Input: part model. Units: mm. Frame: model coordinates. Face numbers are marked on the shaded views. Coordinates: 2 decimals unless noted, no trailing zeros. Loops run counter-clockwise (first coordinate to the right, second up) from the corner with the lowest first, then second, coordinate; pieces in that order, holes last. Notation, with made-up numbers: M -32.5,16 L -4.5,16 A30 ccw -4.5,40 Z; hole C 4,44.25 d6. An arc over 180 degrees is marked long. Use a Markdown table: item, result. Add a question column.
1. Section A-A on z = -31.5. Output: boundary loops of the cut face in (x, y).
2. Line query: L1, parallel to Z at x = 0, y = -244.85; L2, parallel to Z at x = 96, y = -150; L3, parallel to X at y = -150, z = -8. Output: solid intervals per line, ascending. Write a range as [from, to].
3. Draft query along Y for the marked faces 1 and 2. Return one class per face: +Y half, -Y half, draft (parallel to the pull), parting line (faces both ways), or undercut.
4. Pin query (flat end, axial travel): pin 1 (1.5 mm diameter, centred on y = -114.5, z = -52.5, fed in from +X); pin 2 (10 mm diameter, centred on y = -105, z = -14, fed in from -X); pin 3 (3.5 mm diameter, centred on y = -150, z = 8, fed in from +X); pin 4 (3 mm diameter, centred on x = -8, z = -43, fed in from -Y). Return the tip coordinate at first contact, or that it passes through.
```python
from build123d import *

# Parameters (mm, degrees)
SKETCH051_R                 = 2.8
EXTRUDE033_DEPTH            = 20
CYLINDER153_R               = 2.13
CYLINDER153_DEPTH           = 300
CYLINDER154_R               = 2.13
CYLINDER154_DEPTH           = 300
TUBE008_R                   = 98
TUBE008_R_2                 = 94
TUBE008_DEPTH               = 65
SKETCH050_R                 = 98
SKETCH050_R_2               = 76
EXTRUDE032_DEPTH            = 5
FILLET005_R                 = 3
TUBE007_R                   = 98
TUBE007_R_2                 = 95
TUBE007_DEPTH               = 3
CYLINDER150_R               = 2.13
CYLINDER150_DEPTH           = 300
CYLINDER150_ROLL_ANGLE      = 90
CYLINDER150_PLACEMENT_ANGLE = 45
CYLINDER149_R               = 2.13
CYLINDER149_DEPTH           = 300
CYLINDER149_ROLL_ANGLE      = 90
CYLINDER149_PLACEMENT_ANGLE = -45
CYLINDER147_R               = 2.13
CYLINDER147_DEPTH           = 300
CYLINDER148_R               = 2.13
CYLINDER148_DEPTH           = 300
CYLINDER139_R               = 2.13
CYLINDER139_DEPTH           = 300
CYLINDER140_R               = 2.13
CYLINDER140_DEPTH           = 300
TUBE002_R                   = 98
TUBE002_R_2                 = 94
TUBE002_DEPTH               = 80
FILLET006_R                 = 3


with BuildPart() as m4heatsetvercuts005:
    # Sketch051 → Extrude033 (new body)
    with BuildSketch(Plane.XY):
        with Locations((0, -68)):
            Circle(SKETCH051_R)
        with Locations((82, -150)):
            Circle(SKETCH051_R)
        with Locations((0, -232)):
            Circle(SKETCH051_R)
        with Locations((-82, -150)):
            Circle(SKETCH051_R)
    extrude(amount=EXTRUDE033_DEPTH)


with BuildPart() as m4heatsetvercuts005_1:
    # Extrude033 placement: moved
    add(m4heatsetvercuts005.part.moved(Location((0, 0, -193))))


with BuildPart() as cylinder153:
    # Cylinder153 → Cylinder153 (new body)
    with BuildSketch(Plane(origin=(0, 0, 90), x_dir=(1, 0, 0), z_dir=(0, -1, 0))):
        Circle(CYLINDER153_R)
    extrude(amount=CYLINDER153_DEPTH)


with BuildPart() as m4cuts016:
    # Cylinder154 → Cylinder154 (new body)
    with BuildSketch(Plane(origin=(-150, -150, 90), x_dir=(0, 1, 0), z_dir=(1, 0, 0))):
        Circle(CYLINDER154_R)
    extrude(amount=CYLINDER154_DEPTH)

    # Fusion099: union Cylinder153
    add(cylinder153.part)


with BuildPart() as m4cuts016_1:
    # Fusion099 placement: moved
    add(m4cuts016.part.moved(Location((0, 0, -321))))


with BuildPart() as tube008:
    # Tube008 → Tube008 (new body)
    with BuildSketch(Plane(origin=(0, -150, -125), x_dir=(1, 0, 0), z_dir=(0, 0, 1))):
        Circle(TUBE008_R)
        Circle(TUBE008_R_2, mode=Mode.SUBTRACT)
    extrude(amount=TUBE008_DEPTH)


with BuildPart() as level5s003:
    # Sketch050 → Extrude032 (new body)
    with BuildSketch(Plane.XY):
        with Locations((0, -150)):
            Circle(SKETCH050_R)
        with Locations((0, -150)):
            Circle(SKETCH050_R_2, mode=Mode.SUBTRACT)
    extrude(amount=EXTRUDE032_DEPTH)


with BuildPart() as level5s003_1:
    # Extrude032 placement: moved
    add(level5s003.part.moved(Location((0, 0, -65))))

    # Fusion098: union Tube008
    add(tube008.part)


with BuildPart() as level5s003_2:
    # Fusion098 placement: moved
    add(level5s003_1.part.moved(Location((0, 0, -125))))

    # Cut050: cut m4Cuts016
    add(m4cuts016_1.part, mode=Mode.SUBTRACT)

    # Cut051: cut m4HeatSetVerCuts005
    add(m4heatsetvercuts005_1.part, mode=Mode.SUBTRACT)

    # Fillet005
    fillet005_edges = [level5s003_2.edges().sort_by_distance(p)[0] for p in [
        (-98, -150, -185),
        (-98, -150, -250),
        (-94, -150, -190),
    ]]
    fillet(fillet005_edges, radius=FILLET005_R)


with BuildPart() as obj1:
    # Tube007 → Tube007 (new body)
    with BuildSketch(Plane(origin=(0, -150, -188), x_dir=(1, 0, 0), z_dir=(0, 0, 1))):
        Circle(TUBE007_R)
        Circle(TUBE007_R_2, mode=Mode.SUBTRACT)
    extrude(amount=TUBE007_DEPTH)

    # Cut052: cut level5s003
    add(level5s003_2.part, mode=Mode.SUBTRACT)


with BuildPart() as obj1_1:
    # Cut052 placement: moved
    add(obj1.part.moved(Location((0, 0, 125.25))))


with BuildPart() as cylinder150:
    # Cylinder150 → Cylinder150 (new body)
    with BuildSketch(Plane.XY):
        Circle(CYLINDER150_R)
    extrude(amount=CYLINDER150_DEPTH)


with BuildPart() as cylinder150_1:
    # Cylinder150 roll: moved
    add(cylinder150.part.rotate(Axis((0, 0, 0), (1, 0, 0)), CYLINDER150_ROLL_ANGLE))


with BuildPart() as cylinder150_2:
    # Cylinder150 placement: moved
    add(cylinder150_1.part.moved(Location((-106.066017, -43.933983, 90))).rotate(Axis((-106.066017, -43.933983, 90), (0, 0, 1)), CYLINDER150_PLACEMENT_ANGLE))


with BuildPart() as m4cuts013:
    # Cylinder149 → Cylinder149 (new body)
    with BuildSketch(Plane.XY):
        Circle(CYLINDER149_R)
    extrude(amount=CYLINDER149_DEPTH)


with BuildPart() as m4cuts013_1:
    # Cylinder149 roll: moved
    add(m4cuts013.part.rotate(Axis((0, 0, 0), (1, 0, 0)), CYLINDER149_ROLL_ANGLE))


with BuildPart() as m4cuts013_2:
    # Cylinder149 placement: moved
    add(m4cuts013_1.part.moved(Location((106.066017, -43.933983, 90))).rotate(Axis((106.066017, -43.933983, 90), (0, 0, 1)), CYLINDER149_PLACEMENT_ANGLE))

    # Fusion093: union Cylinder150
    add(cylinder150_2.part)


with BuildPart() as m4cuts013_3:
    # Fusion093 placement: moved
    add(m4cuts013_2.part.moved(Location((0, 0, -82))))


with BuildPart() as cylinder147:
    # Cylinder147 → Cylinder147 (new body)
    with BuildSketch(Plane(origin=(0, 0, 90), x_dir=(1, 0, 0), z_dir=(0, -1, 0))):
        Circle(CYLINDER147_R)
    extrude(amount=CYLINDER147_DEPTH)


with BuildPart() as m4cuts014:
    # Cylinder148 → Cylinder148 (new body)
    with BuildSketch(Plane(origin=(-150, -150, 90), x_dir=(0, 1, 0), z_dir=(1, 0, 0))):
        Circle(CYLINDER148_R)
    extrude(amount=CYLINDER148_DEPTH)

    # Fusion092: union Cylinder147
    add(cylinder147.part)


with BuildPart() as m4cuts014_1:
    # Fusion092 placement: moved
    add(m4cuts014.part.moved(Location((0, 0, -82))))

    # Fusion094: union m4Cuts013
    add(m4cuts013_3.part)


with BuildPart() as cylinder139:
    # Cylinder139 → Cylinder139 (new body)
    with BuildSketch(Plane(origin=(0, 0, 90), x_dir=(1, 0, 0), z_dir=(0, -1, 0))):
        Circle(CYLINDER139_R)
    extrude(amount=CYLINDER139_DEPTH)


with BuildPart() as m4cuts011:
    # Cylinder140 → Cylinder140 (new body)
    with BuildSketch(Plane(origin=(-150, -150, 90), x_dir=(0, 1, 0), z_dir=(1, 0, 0))):
        Circle(CYLINDER140_R)
    extrude(amount=CYLINDER140_DEPTH)

    # Fusion088: union Cylinder139
    add(cylinder139.part)


with BuildPart() as m4cuts011_1:
    # Fusion088 placement: moved
    add(m4cuts011.part.moved(Location((0, 0, -130))))


with BuildPart() as level003to2s:
    # Tube002 → Tube002 (new body)
    with BuildSketch(Plane(origin=(0, -150, -60), x_dir=(1, 0, 0), z_dir=(0, 0, 1))):
        Circle(TUBE002_R)
        Circle(TUBE002_R_2, mode=Mode.SUBTRACT)
    extrude(amount=TUBE002_DEPTH)

    # Cut044: cut m4Cuts011
    add(m4cuts011_1.part, mode=Mode.SUBTRACT)

    # Cut046: cut m4Cuts014
    add(m4cuts014_1.part, mode=Mode.SUBTRACT)

    # Fusion100: union obj1
    add(obj1_1.part)

    # Fillet006
    fillet006_edges = [level003to2s.edges().sort_by_distance(p)[0] for p in [
        (-98, -150, 20),
    ]]
    fillet(fillet006_edges, radius=FILLET006_R)


solid = level003to2s.part
```
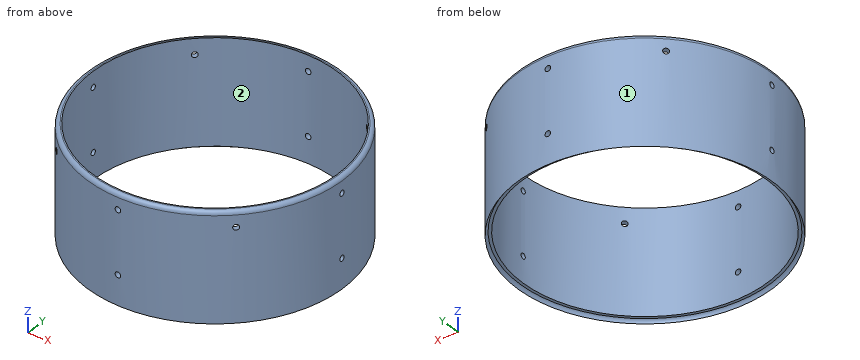
Answers below:
| question | item | result |
|---|---|---|
| 1 | outline | C 0,-150 d196; hole C 0,-150 d188 |
| 2 | L1 | z = [-60, -42.13], [-37.87, 5.87], [10.13, 20] |
| 2 | L2 | z = [-60, -42.13], [-37.87, 5.87], [10.13, 19.83] |
| 2 | L3 | x = [-98, -94], [94, 98] |
| 3 | face 1 | parting line |
| 3 | face 2 | undercut |
| 4 | pin 1 | stops at x = 91.63 |
| 4 | pin 2 | stops at x = -89.47 |
| 4 | pin 3 | passes through |
| 4 | pin 4 | stops at y = -247.78 |
